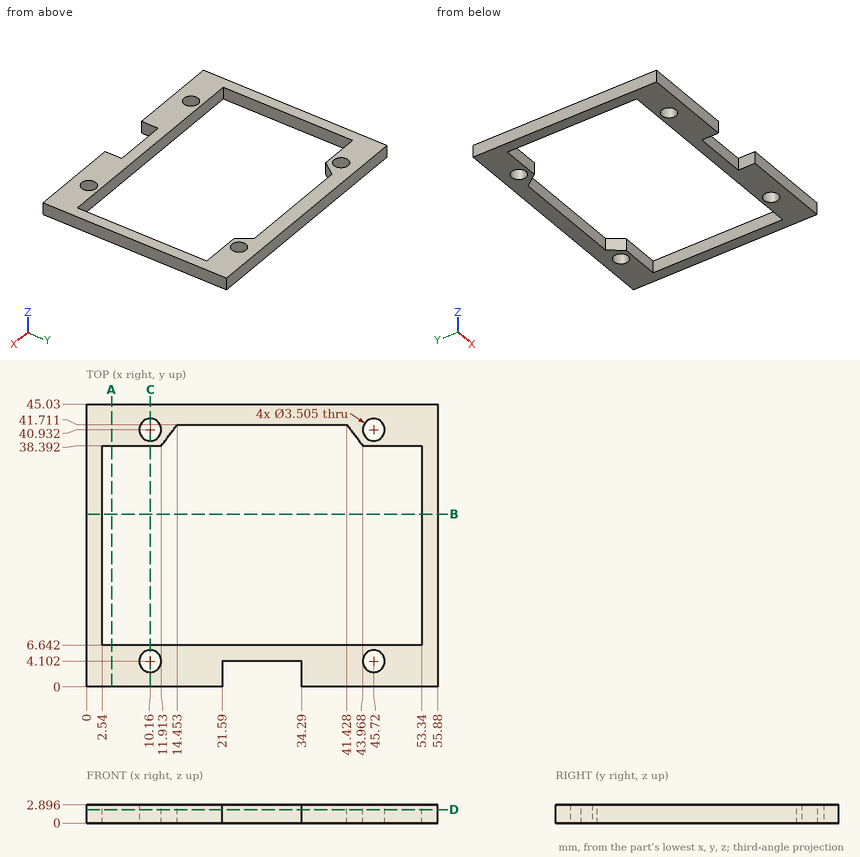
The figure shows three views and two pictorial views of one solid part (mm, origin at its lowest corner). Answer the questions. Give positions to 0.01 mm unless a question says otherwise; leave off trailing zeros. Order: outer loops, then holes, each group sorted by start corner. A loop starts at its lowest first (then second) coordinate and runs counter-clockwise, first axis right, second up. Notation, with made-up numbers: (74.5, -11) -> (117.5, -11) arc R26 ccw to (117.5, 27) -> close; hole circle Ø6 at (-39, 73). An arc over 180 degrees is marked (long way). Answer as CSV lines item,"result". Start each with the question number.
Q1. Given pin 1 (8 mm diameter, centred on x = 14, y = 31.5, fed in from +Z); pin 2 (1.4 mm diameter, centred on x = 25, z = 1.5, fed in from -Y), each flat-ended and moving along its own axis, determine where each tip first touches the part or whether it passes through.
Q2. A cutting plane is placed at C-C (x = 10.16). Count the separate pieces of the cut face and the enclosed holes in it.
Q3. A cutting plane is placed at A-A (x = 4). Determine the outline of the cut face in (y, z) (1 decimal).
Q4. A cutting plane is placed at B-B (y = 27.5). Determine the outline of the cut face in (x, z) (1 decimal).
Q5. A cutting plane is placed at D-D (z = 2.15). Determine the outline of the cut face in (x, y) (1 decimal).
Q6. Find the intervals of material crossed by L1, parallel to X at y = 11.5, z = 0.45; L2, parallel to Y at x = 38, z = 1.4; L3, parallel to Y at x = 49, z = 0.35, in increasing order.
Results found:
1,pin 1,"through"
1,pin 2,"y = 4.1"
2,separate pieces,"4"
2,enclosed holes,"0"
3,outline,"(0, 0) -> (6.6, 0) -> (6.6, 2.9) -> (0, 2.9) -> close; (38.4, 0) -> (45, 0) -> (45, 2.9) -> (38.4, 2.9) -> close"
4,outline,"(0, 0) -> (2.5, 0) -> (2.5, 2.9) -> (0, 2.9) -> close; (53.3, 0) -> (55.9, 0) -> (55.9, 2.9) -> (53.3, 2.9) -> close"
5,outline,"(0, 0) -> (21.6, 0) -> (21.6, 4.1) -> (34.3, 4.1) -> (34.3, 0) -> (55.9, 0) -> (55.9, 45) -> (0, 45) -> close; hole (2.5, 6.6) -> (53.3, 6.6) -> (53.3, 38.4) -> (44, 38.4) -> (41.4, 41.7) -> (14.5, 41.7) -> (11.9, 38.4) -> (2.5, 38.4) -> close; hole circle Ø3.5 at (10.2, 4.1); hole circle Ø3.5 at (10.2, 40.9); hole circle Ø3.5 at (45.7, 4.1); hole circle Ø3.5 at (45.7, 40.9)"
6,L1,"0 to 2.54, 53.34 to 55.88"
6,L2,"0 to 6.64, 41.71 to 45.03"
6,L3,"0 to 6.64, 38.39 to 45.03"
